Check sheet for the modelled part. Datum: model origin and axes. Units: mm. A direction names the side the tool comes from. Give positions to 0.01 mm unless a question says otherwise; leave off trailing zeros. Write each loop counter-clockwise with the first axis right and the second up, starting at its lowest first coordinate (ties: lowest second). Pieces come first, ordered by that corner, then holes. Notation, with made-up numbers: (60, 5) -> (113, 5) arc R27 ccw to (113, 26) -> close; hole circle Ø4 at (75.25, -14). An arc over 180 degrees is marked (long way). Return JSON: item names as keys, results as strings.
from build123d import *

# Parameters (mm, degrees)
CROQUIS1_W                   = 57
CROQUIS1_H                   = 57
SALIENTE_EXTRUIR1_DEPTH      = 113
CROQUIS2_R                   = 5
SALIENTE_EXTRUIR2_DEPTH      = 24
TALADRO_DE_MARGEN_PARA_M51_D = 5.2
CROQUIS8_W                   = 10
CROQUIS8_H                   = 10
CROQUIS8_R                   = 2.6
CORTAR_EXTRUIR1_DEPTH        = 106


with BuildPart() as part:
    # Croquis1 → Saliente-Extruir1 (new body)
    with BuildSketch(Plane(origin=(0, 0, 0), x_dir=(1, 0, 0), z_dir=(0, 1, 0))):
        Rectangle(CROQUIS1_W, CROQUIS1_H)
    extrude(amount=SALIENTE_EXTRUIR1_DEPTH)

    # Croquis2 → Saliente-Extruir2 (add)
    with BuildSketch(Plane(origin=(0, 0, 0), x_dir=(-1, 0, 0), z_dir=(0, -1, 0))):
        with Locations(Location((0, 0, 0), (0, 0, 90))):
            Circle(CROQUIS2_R)
    extrude(amount=SALIENTE_EXTRUIR2_DEPTH)

    # Taladro de margen para M51 (through all)
    with Locations(Plane(origin=(0, 0, 0), x_dir=(-1, 0, 0), z_dir=(0, -1, 0))):
        with Locations((23.5, -23.5), (-23.5, -23.5), (-23.5, 23.5), (23.5, 23.5)):
            Hole(TALADRO_DE_MARGEN_PARA_M51_D / 2)

    # Croquis8 → Cortar-Extruir1 (cut)
    # profile 1 of 6: a face of its own
    with BuildSketch(Plane(origin=(0, 113, 0), x_dir=(1, 0, 0), z_dir=(0, 1, 0))):
        with Locations((-23.5, -23.5)):
            Rectangle(CROQUIS8_W, CROQUIS8_H)
        with Locations(Location((-23.5, -23.5, 0), (0, 0, 90))):
            Circle(CROQUIS8_R, mode=Mode.SUBTRACT)
    # profile 2 of 6: a face of its own
    with BuildSketch(Plane(origin=(0, 113, 0), x_dir=(1, 0, 0), z_dir=(0, 1, 0))):
        with Locations((23.5, -23.5)):
            Rectangle(CROQUIS8_W, CROQUIS8_H)
        with Locations(Location((23.5, -23.5, 0), (0, 0, 90))):
            Circle(CROQUIS8_R, mode=Mode.SUBTRACT)
    # profile 3 of 6: a face of its own
    with BuildSketch(Plane(origin=(0, 113, 0), x_dir=(1, 0, 0), z_dir=(0, 1, 0))):
        with Locations(Location((23.5, -23.5, 0), (0, 0, 90))):
            Circle(CROQUIS8_R)
    # profile 4 of 6: a face of its own
    with BuildSketch(Plane(origin=(0, 113, 0), x_dir=(1, 0, 0), z_dir=(0, 1, 0))):
        with Locations((-23.5, 23.5)):
            Rectangle(CROQUIS8_W, CROQUIS8_H)
        with Locations(Location((-23.5, 23.5, 0), (0, 0, 90))):
            Circle(CROQUIS8_R, mode=Mode.SUBTRACT)
    # profile 5 of 6: a face of its own
    with BuildSketch(Plane(origin=(0, 113, 0), x_dir=(1, 0, 0), z_dir=(0, 1, 0))):
        with Locations(Location((-23.5, 23.5, 0), (0, 0, 90))):
            Circle(CROQUIS8_R)
    # profile 6 of 6: a face of its own
    with BuildSketch(Plane(origin=(0, 113, 0), x_dir=(1, 0, 0), z_dir=(0, 1, 0))):
        with Locations((23.5, 23.5)):
            Rectangle(CROQUIS8_W, CROQUIS8_H)
    extrude(amount=-CORTAR_EXTRUIR1_DEPTH, mode=Mode.SUBTRACT)


solid = part.part
(1) Set-up check for faces 4 (the flat face through (-24, 61, -18.5)), 5 (the flat face through (21, 7, 26)), 6 (the cylindrical face through (24.9, 3.55, -25.69)), 7 (the flat face through (21, 7, -21)), 8 (the flat face through (-24, 61, 18.5)): record each of +Z, -Z, +X, -X, +Y, -Y from which the full face is reachable in a straight line by a thin tool's end or side.
Reply:
{"face 4": "-Z, -X, +Y", "face 5": "+Z, +X, +Y", "face 6": "+Y, -Y", "face 7": "-Z, +X, +Y", "face 8": "+Z, -X, +Y"}
(2) Depth check by flat-ended pin: pin 1 Ø1 at (x, z) = (0, -19.5) entering from -Y; pin 2 Ø3 at (x, y) = (-23.5, 85.5) entering from -Z; pin 3 Ø3 at (x, z) = (23.5, 21.5) entering from +Y; pin 4 Ø4 at (x, z) = (-23.5, 23.5) entering from -Y. Enter the tip coordinate at first touch or a pass-through.
Reply:
{"pin 1": "y = 0", "pin 2": "z = -18.5", "pin 3": "y = 7", "pin 4": "through"}
(3) Cross-section at B-B on z = -23.5. Enter the section's corners in (x, y).
Reply:
{"outline": "(-28.5, 0) -> (-26.1, 0) -> (-26.1, 7) -> (-28.5, 7) -> close; (-20.9, 0) -> (20.9, 0) -> (20.9, 7) -> (18.5, 7) -> (18.5, 113) -> (-18.5, 113) -> (-18.5, 7) -> (-20.9, 7) -> close; (26.1, 0) -> (28.5, 0) -> (28.5, 7) -> (26.1, 7) -> close"}
(4) Cross-section at D-D on y = 102.5. Enter the section's corners in (x, z), then the cut area to 3 significant figures.
Reply:
{"outline": "(-28.5, -18.5) -> (-18.5, -18.5) -> (-18.5, -28.5) -> (18.5, -28.5) -> (18.5, -18.5) -> (28.5, -18.5) -> (28.5, 18.5) -> (18.5, 18.5) -> (18.5, 28.5) -> (-18.5, 28.5) -> (-18.5, 18.5) -> (-28.5, 18.5) -> close", "area": "2,850 mm^2"}
(5) Thickness scan on L1, parallel to X at y = 3.25, z = -23.5; L2, parallel to Y at x = -2, z = -24. Record the ranges inside material, lowest first.
Reply:
{"L1": "-28.5 to -26.1, -20.9 to 20.9, 26.1 to 28.5", "L2": "0 to 113"}
(6) Cross-section at C-C on z = 0. Enter the section's corners in (x, y), then the cut area to 3 significant figures.
Reply:
{"outline": "(-28.5, 0) -> (-5, 0) -> (-5, -24) -> (5, -24) -> (5, 0) -> (28.5, 0) -> (28.5, 113) -> (-28.5, 113) -> close", "area": "6,680 mm^2"}
(7) Cross-section at A-A on x = 23.5. Enter the section's corners in (y, z), then the cut area to 3 significant figures.
Reply:
{"outline": "(0, -28.5) -> (7, -28.5) -> (7, -26.1) -> (0, -26.1) -> close; (0, -20.9) -> (7, -20.9) -> (7, -18.5) -> (113, -18.5) -> (113, 18.5) -> (7, 18.5) -> (7, 20.9) -> (0, 20.9) -> close; (0, 26.1) -> (7, 26.1) -> (7, 28.5) -> (0, 28.5) -> close", "area": "4,250 mm^2"}
(8) Release check for a two-part mould opening along X. For faces 1 (the flat face through (0, 56, 28.5)), 2 (the cylindrical face through (-4.88, -11.83, 1.08)), 3 (the cylindrical face through (-22.1, 3.55, 21.31)) record: pulls with the +X half, pulls with the -X half, needs draft (parallel to the pull), parting line crosses it, or undercut.
Reply:
{"face 1": "needs draft", "face 2": "parting line crosses it", "face 3": "undercut"}
